Autodesk Fusion 360 part; units mm, degrees
sketch "Sketch1" plane through (0, 0, 0) normal (0, 0, 1) x (1, 0, 0)
  line L0 (1.8764, -3.25) -> (3.7528, 0)
  line L1 (3.7528, 0) -> (1.8764, 3.25)
  line L2 (1.8764, 3.25) -> (-1.8764, 3.25)
  line L3 (-1.8764, 3.25) -> (-3.7528, 0)
  line L4 (-3.7528, 0) -> (-1.8764, -3.25)
  line L5 (-1.8764, -3.25) -> (1.8764, -3.25)
  circle A0 centre (0, 0) radius 4.75
  dimension "d1" = 3.25
  dimension "d2" = 9.5
extrude "Extrude1" add sketch "Sketch1" along normal blind 13
sketch "Sketch2" plane through (0, 0, 13) normal (0, 0, 1) x (-1, 0, 0)
  line L0 (-1.8764, 3.25) -> (1.8764, 3.25)
  line L1 (1.8764, 3.25) -> (3.7528, 0)
  line L2 (3.7528, 0) -> (1.8764, -3.25)
  line L3 (1.8764, -3.25) -> (-1.8764, -3.25)
  line L4 (-1.8764, -3.25) -> (-3.7528, 0)
  line L5 (-3.7528, 0) -> (-1.8764, 3.25)
  circle A0 centre (0, 0) radius 4.75
extrude "Extrude2" add sketch "Sketch2" along normal blind 1 contours L0 L1 L2 L3 L4 L5 | A0
sketch "Sketch3" plane through (0, 0, 14) normal (0, 0, 1) x (-1, 0, 0)
  circle A0 centre (0, 0) radius 4.75
  circle A1 centre (0, 0) radius 2.4
  dimension "d7" = 4.8
extrude "Extrude3" add sketch "Sketch3" along normal blind 16.8
Work out the finished part from the listing and answer in its coordinate system (mm). A direction names the side the tool comes from. Give positions to 0.01 mm unless a question says otherwise; leave off trailing zeros. Order: outer loops, then holes, each group sorted by start corner. A loop starts at its lowest first (then second) coordinate and runs counter-clockwise, first axis right, second up. Notation, with made-up numbers: (52, 32.5) - (99, 32.5) arc R16 cw to (99, 37.5) - close; hole circle Ø4 at (85.25, 86.25). An arc over 180 degrees is marked (long way). One line per item, written item: value. Start each with the question number.
1. Section C-C, the plane z = 15.5 is taken. Write down the section's boundary in (x, y).
2. Consider line 1 (X direction, y = 0, z = 21.75); line 2 (Z direction, x = 2.75, y = 0.5). Determine where each line is inside the solid, lowest interval first.
3. Section B-B, the plane y = -1.5 is taken. Write down the section's boundary in (x, z).
4. Each of these flat-tipped pins is pushed along its axis until it touches: pin 1 Ø4 at (x, y) = (-0.5, -0.5) entering from +Z; pin 2 Ø2 at (y, z) = (-1.5, 26) entering from -X; pin 3 Ø1 at (y, z) = (-2, 11.5) entering from -X; pin 4 Ø2 at (x, z) = (3, 17) entering from +Y. Where does it stop, or does it pass through?
5. Which of the six approach directions +Z, -Z, +X, -X, +Y, -Y give full straight-line access (tool end or side, diameter ignored) to faces 3 (the face through (-1.29, 2.024, 22.282)), 4 (the face through (-2, 2, 30.8)), 5 (the face through (-2.8, 1.65, 6.41))?
6. Section A-A, the plane z = 5 is taken. Write down the section's boundary in (x, y).
7. For a pull along X with two mould halves and no side action, classify faces 1 (the face through (0, -3.25, 6)), 2 (the face through (3, -2, 0)) as released by +X, released by -X, zero draft, split by the parting line, or undercut.
Filled sheet:
1. outline: circle Ø9.5 at (0, 0); hole circle Ø4.8 at (0, 0)
2. line 1: -4.75 to -2.4, 2.4 to 4.75
2. line 2: 13 to 30.8
3. outline: (-4.51, 0) - (-2.89, 0) - (-2.89, 13) - (2.89, 13) - (2.89, 0) - (4.51, 0) - (4.51, 30.8) - (1.87, 30.8) - (1.87, 14) - (-1.87, 14) - (-1.87, 30.8) - (-4.51, 30.8) - close
4. pin 1: z = 30.8
4. pin 2: x = -4.72
4. pin 3: x = -4.51
4. pin 4: y = 4.31
5. face 3: +Z
5. face 4: +Z, +X, -X, +Y, -Y
5. face 5: -Z
6. outline: circle Ø9.5 at (0, 0); hole (-3.75, 0) - (-1.88, -3.25) - (1.88, -3.25) - (3.75, 0) - (1.88, 3.25) - (-1.88, 3.25) - close
7. face 1: undercut
7. face 2: zero draft
